Geometry: final body of the model. Coordinates: model frame, mm. Give positions to 0.01 mm unless a question says otherwise; leave off trailing zeros. Write each loop counter-clockwise with the first axis right and the second up, starting at its lowest first coordinate (ties: lowest second). Pieces come first, ordered by that corner, then holes.
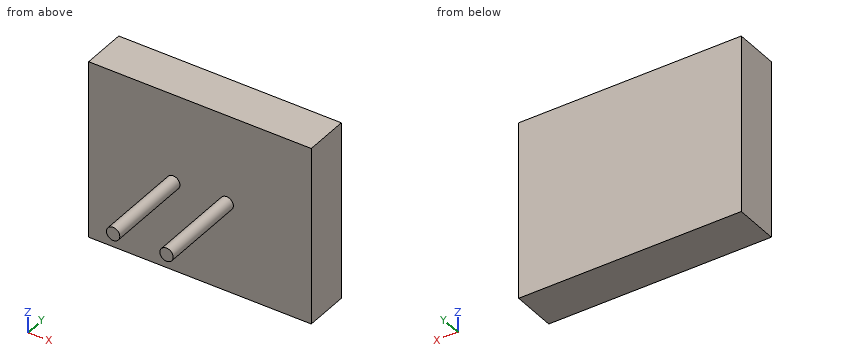
from build123d import *

# Parameters (mm, degrees)
SZKIC1_W                    = 50
SZKIC1_H                    = 10
DODANIE_WYCI_GNI_CIE1_DEPTH = 40
SZKIC2_R                    = 1.5
DODANIE_WYCI_GNI_CIE2_DEPTH = 20


with BuildPart() as part:
    # Szkic1 → Dodanie-wyciągnięcie1 (new body)
    with BuildSketch(Plane.XY):
        Rectangle(SZKIC1_W, SZKIC1_H)
    extrude(amount=DODANIE_WYCI_GNI_CIE1_DEPTH)

    # Szkic2 → Dodanie-wyciągnięcie2 (add)
    with BuildSketch(Plane.XZ.offset(5)):
        with Locations(Location((-6, 20, 0), (0, 0, 90))):
            Circle(SZKIC2_R)
        with Locations(Location((6, 20, 0), (0, 0, 90))):
            Circle(SZKIC2_R)
    extrude(amount=DODANIE_WYCI_GNI_CIE2_DEPTH)


solid = part.part
Q1. Ray query, line 1 along Y through (x, z) = (-5, 34.5). Return the intervals inside material, ascending.
Filled sheet:
line 1: y = -5 to 5
Q2. Section C-C on x = -6. Output: boundary loops of the cut face in (y, z).
Filled sheet:
outline: (-25, 18.5) - (-5, 18.5) - (-5, 0) - (5, 0) - (5, 40) - (-5, 40) - (-5, 21.5) - (-25, 21.5) - close
Q3. Section B-B on y = -18. Output: boundary loops of the cut face in (x, z), plus the area to 3 significant figures.
Filled sheet:
outline: circle Ø3 at (-6, 20); circle Ø3 at (6, 20)
area: 14.1 mm2
Q4. Pin query (flat end, axial travel): P1, Ø10, axis at x = -10, y = -9, coming from the +Z side. Return the tip coordinate at first contact, or that it passes through.
Filled sheet:
P1: stops at z = 40
Q5. Section D-D on x = -14. Output: boundary loops of the cut face in (y, z), plus the area to 3 significant figures.
Filled sheet:
outline: (-5, 0) - (5, 0) - (5, 40) - (-5, 40) - close
area: 400 mm2
Q6. Section A-A on z = 20. Output: boundary loops of the cut face in (x, y).
Filled sheet:
outline: (-25, -5) - (-7.5, -5) - (-7.5, -25) - (-4.5, -25) - (-4.5, -5) - (4.5, -5) - (4.5, -25) - (7.5, -25) - (7.5, -5) - (25, -5) - (25, 5) - (-25, 5) - close
